```python
from build123d import *

# Parameters (mm, degrees)
SKETCH_1_W          = 60
SKETCH_1_H          = 45
EXTRUDE_1_DEPTH     = 2
FILLET_1_R          = 4
SKETCH_2_R          = 1.5
CUT_EXTRUDE_1_DEPTH = 2
SKETCH_3_R          = 1.6
CUT_EXTRUDE_2_DEPTH = 2
SKETCH_4_R          = 6.25
CUT_EXTRUDE_3_DEPTH = 2


with BuildPart() as part:
    # 草图1 → 凸台-拉伸1 (new body)
    with BuildSketch(Plane.XY):
        with Locations((30, 22.5)):
            Rectangle(SKETCH_1_W, SKETCH_1_H)
    extrude(amount=EXTRUDE_1_DEPTH)

    # 圆角1
    fillet_1_edges = [part.edges().sort_by_distance(p)[0] for p in [
        (0, 45, 1),
        (60, 45, 1),
        (60, 0, 1),
        (0, 0, 1),
    ]]
    fillet(fillet_1_edges, radius=FILLET_1_R)

    # 草图2 → 切除-拉伸1 (cut)
    with BuildSketch(Plane(origin=(0, 0, 0), x_dir=(-1, 0, 0), z_dir=(0, 0, -1))):
        with Locations((-39, 4)):
            Circle(SKETCH_2_R)
        with Locations((-21, 4)):
            Circle(SKETCH_2_R)
    extrude(amount=-CUT_EXTRUDE_1_DEPTH, mode=Mode.SUBTRACT)

    # 草图3 → 切除-拉伸2 (cut)
    with BuildSketch(Plane.XY.offset(2)):
        with Locations((5.7, 36.9)):
            Circle(SKETCH_3_R)
        with Locations((5.7, 27.1)):
            Circle(SKETCH_3_R)
        with Locations((54.3, 36.9)):
            Circle(SKETCH_3_R)
        with Locations((54.3, 27.1)):
            Circle(SKETCH_3_R)
    extrude(amount=-CUT_EXTRUDE_2_DEPTH, mode=Mode.SUBTRACT)

    # 草图4 → 切除-拉伸3 (cut)
    with BuildSketch(Plane.XY.offset(2)):
        with Locations((20, 32)):
            Circle(SKETCH_4_R)
    extrude(amount=-CUT_EXTRUDE_3_DEPTH, mode=Mode.SUBTRACT)


solid = part.part
```
The listing builds one solid part. Answer for the finished solid, in the listing's coordinates (mm). Round coordinates to 2 decimals unless told otherwise and drop trailing zeros. Order: outer loops, then holes, each group sorted by start corner. A loop starts at its lowest first (then second) coordinate and runs counter-clockwise, first axis right, second up. Notation, with made-up numbers: (12.5, -18) - (38.5, -18) arc R22 ccw to (38.5, 15) - close; hole circle Ø1 at (81.5, 60). An arc over 180 degrees is marked (long way). Put each result on its own line as item: value. Start each with the question number.
(1) Determine the mould class of faces 1 (the cylindrical face through (15.39, 36.22, 1.01)), 2 (the flat face through (30, 45, 1)), 3 (the cylindrical face through (1.141, 43.797, 1.014)) for opening direction X: released by +X, released by -X, zero draft, split by the parting line, or undercut.
(2) Find section A-A (x = 54.3). Give the vertices of the cut face in (y, z).
(3) Straight lines are drawn through the part: probe 1 along Y at (x, z) = (54.3, 0.6); probe 2 along Y at (x, z) = (39, 0.7); probe 3 along Y at (x, z) = (21, 1). For each, find the intervals that lie inside material, in ascending order. Write a range as from..to.
(4) Find section C-C (z = 1.65). Give the vertices of the cut face in (x, y), plus the area to 3 significant figures.
(5) Find section B-B (y = 32). Give the vertices of the cut face in (x, z).
(6) Find section D-D (x = 39). Give the vertices of the cut face in (y, z), plus the area to 3 significant figures.
(7) Given P1, Ø3.5, axis at x = 39, y = 4, coming from the +Z side, flat-ended and moving along its own axis, determine where the tip first touches the part or whether it passes through.
Reply:
1. face 1: undercut
1. face 2: zero draft
1. face 3: released by -X
2. outline: (0, 0) - (25.5, 0) - (25.5, 2) - (0, 2) - close; (28.7, 0) - (35.3, 0) - (35.3, 2) - (28.7, 2) - close; (38.5, 0) - (45, 0) - (45, 2) - (38.5, 2) - close
3. probe 1: 0..25.5, 28.7..35.3, 38.5..45
3. probe 2: 0..2.5, 5.5..45
3. probe 3: 0..2.5, 5.5..25.83, 38.17..45
4. outline: (0, 4) arc R4 ccw to (4, 0) - (56, 0) arc R4 ccw to (60, 4) - (60, 41) arc R4 ccw to (56, 45) - (4, 45) arc R4 ccw to (0, 41) - close; hole circle Ø3.2 at (5.7, 27.1); hole circle Ø3.2 at (5.7, 36.9); hole circle Ø12.5 at (20, 32); hole circle Ø3 at (21, 4); hole circle Ø3 at (39, 4); hole circle Ø3.2 at (54.3, 27.1); hole circle Ø3.2 at (54.3, 36.9)
4. area: 2,520 mm^2
5. outline: (0, 0) - (13.75, 0) - (13.75, 2) - (0, 2) - close; (26.25, 0) - (60, 0) - (60, 2) - (26.25, 2) - close
6. outline: (0, 0) - (2.5, 0) - (2.5, 2) - (0, 2) - close; (5.5, 0) - (45, 0) - (45, 2) - (5.5, 2) - close
6. area: 84.0 mm^2
7. P1: z = 2
